```python
from build123d import *

# Parameters (mm, degrees)
F0_R     = 44.45
F1_DEPTH = 6.35
F2_R     = 16.7386
F3_DEPTH = 6.35
F10_D    = 4.4958
F11_D    = 4.4958
F12_D    = 4.4958
F13_D    = 4.4958
F14_D    = 4.4958
F15_D    = 4.4958


with BuildPart() as f1:
    # F0 (on Top) → F1 (new body)
    with BuildSketch(Plane.XY):
        Circle(F0_R)
    extrude(amount=F1_DEPTH)

    # F2 (on face) → F3 (cut)
    with BuildSketch(Plane.XY.offset(6.35)):
        Circle(F2_R)
    extrude(amount=-F3_DEPTH, mode=Mode.SUBTRACT)

    # F10 (through all)
    with Locations(Plane(origin=(0, 0, 0), x_dir=(1, 0, 0), z_dir=(0, 0, -1))):
        with Locations((0, -23.7994737715)):
            Hole(F10_D / 2)

    # F11 (through all)
    with Locations(Plane(origin=(0, 0, 0), x_dir=(1, 0, 0), z_dir=(0, 0, -1))):
        with Locations((-20.6213220954, -11.9066275656)):
            Hole(F11_D / 2)

    # F12 (through all)
    with Locations(Plane(origin=(0, 0, 0), x_dir=(1, 0, 0), z_dir=(0, 0, -1))):
        with Locations((20.6105131656, -11.9145931676)):
            Hole(F12_D / 2)

    # F13 (through all)
    with Locations(Plane(origin=(0, 0, 0), x_dir=(1, 0, 0), z_dir=(0, 0, -1))):
        with Locations((-20.6335756557, 11.8970761348)):
            Hole(F13_D / 2)

    # F14 (through all)
    with Locations(Plane(origin=(0, 0, 0), x_dir=(1, 0, 0), z_dir=(0, 0, -1))):
        with Locations((20.6222459674, 11.9062252343)):
            Hole(F14_D / 2)

    # F15 (through all)
    with Locations(Plane(origin=(0, 0, 0), x_dir=(1, 0, 0), z_dir=(0, 0, -1))):
        with Locations((0, 23.8109349498)):
            Hole(F15_D / 2)


solid = f1.part
```
Input: part model. Units: mm. Frame: model coordinates. Coordinates: 2 decimals unless noted, no trailing zeros. Write each loop counter-clockwise with the first axis right and the second up, starting at its lowest first coordinate (ties: lowest second). Pieces come first, ordered by that corner, then holes. Notation, with made-up numbers: (74.25, -23) -> (85.25, -23) arc R20 cw to (85.25, 0) -> close; hole circle Ø1 at (15.25, 35.25). An arc over 180 degrees is marked (long way). Answer as a JSON object with one key per item and string values.
1. Section D-D on z = 5.25. Return the cut outline in (x, y).
Result set:
{"outline": "circle Ø88.9 at (0, 0); hole circle Ø4.5 at (-20.63, -11.9); hole circle Ø4.5 at (-20.62, 11.91); hole circle Ø33.48 at (0, 0); hole circle Ø4.5 at (0, -23.81); hole circle Ø4.5 at (0, 23.8); hole circle Ø4.5 at (20.61, 11.91); hole circle Ø4.5 at (20.62, -11.91)"}
2. Section A-A on y = 0. Return the cut outline in (x, z).
Result set:
{"outline": "(-44.45, 0) -> (-16.74, 0) -> (-16.74, 6.35) -> (-44.45, 6.35) -> close; (16.74, 0) -> (44.45, 0) -> (44.45, 6.35) -> (16.74, 6.35) -> close"}
3. Mould query, pull axis Y, two halves, no side actions, for faces 1 (the face through (-22.698, 12.768, 3.219)), 2 (the face through (42.397, 13.352, 3.131)), 3 (the face through (-1, -19, 0)), 4 (the face through (19.41, -13.8, 3.22)). Classes: released by +Y, released by -Y, zero draft, split by the parting line, or undercut.
Result set:
{"face 1": "undercut", "face 2": "split by the parting line", "face 3": "zero draft", "face 4": "undercut"}
4. Section B-B on x = 0. Return the cut outline in (y, z).
Result set:
{"outline": "(-44.45, 0) -> (-26.06, 0) -> (-26.06, 6.35) -> (-44.45, 6.35) -> close; (-21.56, 0) -> (-16.74, 0) -> (-16.74, 6.35) -> (-21.56, 6.35) -> close; (16.74, 0) -> (21.55, 0) -> (21.55, 6.35) -> (16.74, 6.35) -> close; (26.05, 0) -> (44.45, 0) -> (44.45, 6.35) -> (26.05, 6.35) -> close"}
5. Material intervals for line 1 (Y direction, x = -1.5, z = 5.75); line 2 (X direction, y = 11.5, z = 1.5); line 3 (Y direction, x = -14, z = 1.75) (3 decimals), sorted ascending. Write a range as from..to.
Result set:
{"line 1": "y = -44.42..-25.49, -22.14..-16.67, 16.67..22.13, 25.47..44.42", "line 2": "x = -42.94..-22.83, -18.41..-12.16, 12.16..18.4, 22.82..42.94", "line 3": "y = -42.188..-9.175, 9.175..42.188"}
6. First-contact query: P1, Ø3.5, axis at x = 0, y = 23.8, coming from the +Z side; P2, Ø1, axis at x = 2, z = 5, coming from the +Y side. Flat tips, straight axial feed; report the tip coordinate or a pass-through.
Result set:
{"P1": "passes through", "P2": "stops at y = 44.42"}
7. Section C-C on x = 21. Return the cut outline in (y, z), then the cut area to 3 significant figures.
Result set:
{"outline": "(-39.18, 0) -> (-14.12, 0) -> (-14.12, 6.35) -> (-39.18, 6.35) -> close; (-9.69, 0) -> (9.7, 0) -> (9.7, 6.35) -> (-9.69, 6.35) -> close; (14.13, 0) -> (39.18, 0) -> (39.18, 6.35) -> (14.13, 6.35) -> close", "area": "441 mm2"}
